The listing builds one solid part. Answer for the finished solid, in the listing's coordinates (mm). Round coordinates to 2 decimals unless told otherwise and drop trailing zeros. Write each loop counter-clockwise with the first axis right and the second up, starting at its lowest first coordinate (ties: lowest second). Pieces come first, ordered by that corner, then holes.
from build123d import *

# Parameters (mm, degrees)
SKETCH1_R           = 2.38125
SKETCH1_R_2         = 1.651
BOSS_EXTRUDE1_DEPTH = 4.445
FILLET1_R           = 1.27


with BuildPart() as part:
    # Sketch1 → Boss-Extrude1 (new body)
    with BuildSketch(Plane.XY):
        with BuildLine():
            Line((0, 5.08), (31.75, 5.08))
            ThreePointArc((31.75, 5.08), (36.83, 0), (31.75, -5.08))
            Line((31.75, -5.08), (0, -5.08))
            ThreePointArc((0, -5.08), (-5.08, 0), (0, 5.08))
        make_face()
        Circle(SKETCH1_R, mode=Mode.SUBTRACT)
        with Locations((31.75, 0)):
            Circle(SKETCH1_R_2, mode=Mode.SUBTRACT)
    extrude(amount=BOSS_EXTRUDE1_DEPTH)

    # Fillet1
    fillet1_edges = [part.edges().sort_by_distance(p)[0] for p in [
        (36.83, 0, 4.445),
        (15.875, 5.08, 4.445),
        (-5.08, 0, 4.445),
        (15.875, 5.08, 0),
        (36.83, 0, 0),
        (15.875, -5.08, 0),
        (-5.08, 0, 0),
        (15.875, -5.08, 4.445),
    ]]
    fillet(fillet1_edges, radius=FILLET1_R)


solid = part.part
1. Given pin 1 (2.5 mm diameter, centred on x = 31.75, y = 0, fed in from -Z), flat-ended and moving along its own axis, determine where the tip first touches the part or whether it passes through.
Geometry says:
pin 1: passes through
2. Straight lines are drawn through the part: line 1 along X through (y, z) = (1.5, 1.9); line 2 along X through (y, z) = (-1.5, 3.5); line 3 along Y through (x, z) = (31.75, 2.8). For each, find the intervals that lie inside material, in ascending order.
Geometry says:
line 1: x = -4.85 to -1.85, 1.85 to 31.06, 32.44 to 36.6
line 2: x = -4.81 to -1.85, 1.85 to 31.06, 32.44 to 36.56
line 3: y = -5.08 to -1.65, 1.65 to 5.08
3. Section B-B on x = 20.5 is taken. Determine the outline of the cut face in (y, z) (3 decimals).
Geometry says:
outline: (-5.08, 1.27) arc R1.27 ccw to (-3.81, 0) - (3.81, 0) arc R1.27 ccw to (5.08, 1.27) - (5.08, 3.175) arc R1.27 ccw to (3.81, 4.445) - (-3.81, 4.445) arc R1.27 ccw to (-5.08, 3.175) - close
4. Section D-D on z = 3.65 is taken. Determine the outline of the cut face in (x, y), plus the area to 3 significant figures.
Geometry says:
outline: (0, -4.99) - (31.75, -4.99) arc R4.99 ccw to (31.75, 4.99) - (0, 4.99) arc R4.99 ccw to start; hole circle Ø4.76 at (0, 0); hole circle Ø3.3 at (31.75, 0)
area: 369 mm2
5. Section A-A on y = 0 is taken. Determine the outline of the cut face in (x, z) (3 decimals), plus the area to 3 significant figures.
Geometry says:
outline: (-5.08, 1.27) arc R1.27 ccw to (-3.81, 0) - (-2.381, 0) - (-2.381, 4.445) - (-3.81, 4.445) arc R1.27 ccw to (-5.08, 3.175) - close; (2.381, 0) - (30.099, 0) - (30.099, 4.445) - (2.381, 4.445) - close; (33.401, 0) - (35.56, 0) arc R1.27 ccw to (36.83, 1.27) - (36.83, 3.175) arc R1.27 ccw to (35.56, 4.445) - (33.401, 4.445) - close
area: 149 mm2
6. For a pull along Y with two mould halves and no side action, classify faces 1 (the face through (30.1, 0.07, 2.19)), 2 (the face through (16, 0, 4.445)), 3 (the face through (16, 5.08, 2)) as released by +Y, released by -Y, zero draft, split by the parting line, or undercut.
Geometry says:
face 1: undercut
face 2: zero draft
face 3: released by +Y
7. Section C-C on z = 1.7 is taken. Determine the outline of the cut face in (x, y), plus the area to 3 significant figures.
Geometry says:
outline: (0, -5.08) - (31.75, -5.08) arc R5.08 ccw to (31.75, 5.08) - (0, 5.08) arc R5.08 ccw to start; hole circle Ø4.76 at (0, 0); hole circle Ø3.3 at (31.75, 0)
area: 377 mm2
